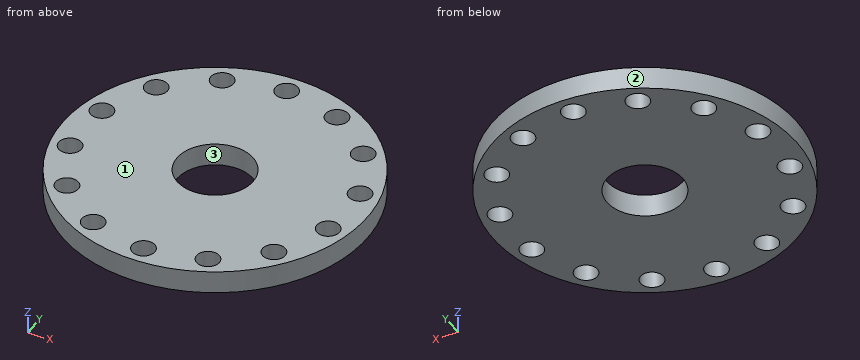
Solid Edge part; units mm, degrees
sketch "Sketch1" plane through (0, 0, 0) normal (0, -1, 0) x (1, 0, 0)
  line L0 (3.75, 0.75) -> (-3.75, 0.75)
  line L1 (-3.75, 0.75) -> (-3.75, -0.75)
  line L2 (-3.75, -0.75) -> (3.75, -0.75)
  line L3 (3.75, -0.75) -> (3.75, 0.75)
revolve "RevolvedProtrusion1" add sketch "Sketch1" angle 360 about axis through (6.25, 0, -3.2815) along (0, 0, 1)
hole "Hole1" at (6.2958, 8.745, -0.75) direction (0, 0, 1) diameter 1.5 end up to next
pattern_circular "Pattern1" count 14 over 360 about axis through (6.25, 0, 0.75) along (0, 0, -1) of "Hole1"
The listing builds one solid part. Answer for the finished solid, in the listing's coordinates (mm). Face numbers are marked on the shaded views. Coordinates: 2 decimals unless noted, no trailing zeros. Loops run counter-clockwise (first coordinate to the right, second up) from the corner with the lowest first, then second, coordinate; pieces in that order, holes last. Notation, with made-up numbers: M 74.25,-2.5 L 88.25,-2.5 A35 ccw 88.25,31.5 Z; hole C 18,10.25 d11. An arc over 180 degrees is marked long. Answer as a JSON object with one key per item and string values. Group by question number.
Item 1: This flat-tipped pin is pushed along its axis until it touches: P1, Ø0.9, axis at x = 6.2, y = -8.74, coming from the -Z side. Where does it stop, or does it pass through?
Item 2: Section D-D (x = 12.75) is taken. Write down the section's boundary in (y, z).
Item 3: Section C-C (y = 7.5) is taken. Write down the section's boundary in (x, z).
Item 4: Determine the mould class of the marked faces 1, 2 and 3 for opening direction Y: +Y half, -Y half, draft (parallel to the pull), parting line (faces both ways), or undercut.
Item 5: Consider L1, parallel to X at y = 0, z = 0.15; L2, parallel to Y at x = 6.5, z = 0.25; L3, parallel to Y at x = 15.25, z = 0.6. Determine where each line is inside the solid, lowest interval first.
Item 6: Section B-B (x = 5) is taken. Write down the section's boundary in (y, z).
Item 7: Section A-A (y = 0) is taken. Write down the section's boundary in (x, z), and give its area (3 significant figures).
Solved:
{
 "1": {"P1": "passes through"},
 "2": {"outline": "M -7.6,-0.75 L -6.17,-0.75 L -6.17,0.75 L -7.6,0.75 Z; M -4.8,-0.75 L 4.76,-0.75 L 4.76,0.75 L -4.8,0.75 Z; M 6.07,-0.75 L 7.6,-0.75 L 7.6,0.75 L 6.07,0.75 Z"},
 "3": {"outline": "M -0.36,-0.75 L 1.86,-0.75 L 1.86,0.75 L -0.36,0.75 Z; M 3.13,-0.75 L 9.43,-0.75 L 9.43,0.75 L 3.13,0.75 Z; M 10.74,-0.75 L 12.86,-0.75 L 12.86,0.75 L 10.74,0.75 Z"},
 "4": {"face 1": "draft", "face 2": "parting line", "face 3": "undercut"},
 "5": {"L1": "x = -3.75 to 3.75, 8.75 to 16.25", "L2": "y = -10 to -9.43, -8.06 to -2.49, 2.49 to 8.02, 9.47 to 10", "L3": "y = -4.36 to -2.56, -1.42 to 1.31, 2.49 to 4.36"},
 "6": {"outline": "M -9.92,-0.75 L -2.17,-0.75 L -2.17,0.75 L -9.92,0.75 Z; M 2.17,-0.75 L 9.92,-0.75 L 9.92,0.75 L 2.17,0.75 Z"},
 "7": {"outline": "M -3.75,-0.75 L 3.75,-0.75 L 3.75,0.75 L -3.75,0.75 Z; M 8.75,-0.75 L 16.25,-0.75 L 16.25,0.75 L 8.75,0.75 Z", "area": "22.5 mm2"}
}
